Check sheet for the modelled part. Datum: model origin and axes. Units: mm. A direction names the side the tool comes from. Give positions to 0.01 mm unless a question says otherwise; leave off trailing zeros. Order: outer loops, then holes, each group sorted by start corner. A loop starts at its lowest first (then second) coordinate and runs counter-clockwise, first axis right, second up. Notation, with made-up numbers: M 38,16 L 76,16 A27 ccw 76,41 Z; hole C 21,4.25 d7. An arc over 180 degrees is marked long. Answer in a Markdown table with one row per item. Add a question column.
from build123d import *

# Parameters (mm, degrees)
F1_DEPTH = 30


with BuildPart() as f1:
    # F0 (on Top) → F1 (new body)
    with BuildSketch(Plane.XY):
        with BuildLine():
            ThreePointArc((0, 10), (2.928932, 2.928932), (10, 0))
            Line((10, 0), (60, 0))
            Line((60, 0), (60, 10))
            Line((60, 10), (30, 10))
            Line((30, 10), (30, 23.99263))
            Line((30, 23.99263), (20, 23.99263))
            Line((20, 23.99263), (20, 40))
            Line((20, 40), (10, 40))
            ThreePointArc((10, 40), (2.928932, 37.071068), (0, 30))
            Line((0, 30), (0, 10))
        make_face()
    extrude(amount=F1_DEPTH)


solid = f1.part
Q1. Thickness scan on probe 1 along X at (y, z) = (9.5, 13.5); probe 2 along X at (y, z) = (11, 28); probe 3 along Y at (x, z) = (33.5, 8). Record the ranges inside material, lowest first.
Q2. Cross-section at B-B (x = 21.5). Record the boundary of the cut face in (y, z), and give its area (3 significant figures).
Q3. Cross-section at C-C (y = 14). Record the boundary of the cut face in (x, z).
Q4. Go/stop test with flat-tipped pins: pin 1 (17.5 mm diameter, centred on y = 32.5, z = 18.5, fed in from +X); pin 2 (10 mm diameter, centred on x = 30, z = 15.5, fed in from +Y). Record where each tip stops, or that it passes through.
Q5. Cross-section at A-A (z = 14). Record the boundary of the cut face in (x, y).
Q6. Tool access check on faces 1 (the flat face through (30, 17, 15)), 2 (the cylindrical face through (2.85, 3.01, 14.79)). Record the directions out of +Z, -Z, +X, -X, +Y, -Y that give a thin tool (end or side, any length) a straight path to the whole face; none if there is none.
Values follow:
| question | item | result |
|---|---|---|
| 1 | probe 1 | 0.01 to 60 |
| 1 | probe 2 | 0 to 30 |
| 1 | probe 3 | 0 to 10 |
| 2 | outline | M 0,0 L 23.99,0 L 23.99,30 L 0,30 Z |
| 2 | area | 720 mm² |
| 3 | outline | M 0,0 L 30,0 L 30,30 L 0,30 Z |
| 4 | pin 1 | x = 30 |
| 4 | pin 2 | y = 23.99 |
| 5 | outline | M 0,10 A10 ccw 10,0 L 60,0 L 60,10 L 30,10 L 30,23.99 L 20,23.99 L 20,40 L 10,40 A10 ccw 0,30 Z |
| 6 | face 1 | +Z, -Z, +X, +Y |
| 6 | face 2 | +Z, -Z, -X, -Y |
